CAD build for the part. Positions are in the model's coordinates, mm. A direction names the side the tool comes from. Give positions to 0.01 mm unless a question says otherwise; leave off trailing zeros. Order: outer loops, then holes, each group sorted by start corner. A loop starts at its lowest first (then second) coordinate and runs counter-clockwise, first axis right, second up. Notation, with made-up numbers: (45.5, 54) -> (63.5, 54) arc R21 ccw to (63.5, 87) -> close; hole circle Ø6 at (14, 67.5). An arc over 180 degrees is marked (long way). Answer as CSV lines item,"result".
```python
from build123d import *

# Parameters (mm, degrees)
PAD002_DEPTH    = 25
SKETCH003_R     = 1.1
SKETCH003_W     = 25
SKETCH003_H     = 10
POCKET_DEPTH    = 5
PAD015_DEPTH    = 20
SKETCH029_R     = 1.65
SKETCH029_W     = 23.5
SKETCH029_H     = 12
POCKET009_DEPTH = 50


with BuildPart() as part:
    # Sketch002 → Pad002 (new body)
    with BuildSketch(Plane.XY):
        Polygon((100, 33), (100, 43), (98, 43), (0, 43), (0, 0), (3, 0), (3, 40), (85.5, 28), (85.5, 40), (98, 40), (98, -20), (100, -20), (100, 31), (103.5, 31), (103.5, 43), (102.3, 43), (102.3, 33), align=None)
    extrude(amount=PAD002_DEPTH)

    # Sketch003 → Pocket (cut)
    with BuildSketch(Plane.YZ):
        with Locations((2, 23)):
            Circle(SKETCH003_R)
        with Locations((2, 2)):
            Circle(SKETCH003_R)
        with Locations((14.5, 23)):
            Circle(SKETCH003_R)
        with Locations((14.5, 2)):
            Circle(SKETCH003_R)
        with Locations((12.5, 12.5)):
            Rectangle(SKETCH003_W, SKETCH003_H)
    extrude(amount=POCKET_DEPTH, mode=Mode.SUBTRACT)

    # Sketch018 → Pad015 (join)
    with BuildSketch(Plane.XZ):
        Polygon((100, 0), (100, -103), (83.5, -103), (83.5, -89), (85.5, -89), (85.5, -101), (98, -101), (98, 0), align=None)
    extrude(amount=PAD015_DEPTH)

    # Sketch029 → Pocket009 (cut)
    with BuildSketch(Plane.XY):
        with Locations((54.956858, 34.491576)):
            Circle(SKETCH029_R)
        with Locations((82.956858, 34.491576)):
            Circle(SKETCH029_R)
        with Locations((68.956858, 34.491576)):
            Rectangle(SKETCH029_W, SKETCH029_H)
    extrude(amount=POCKET009_DEPTH, mode=Mode.SUBTRACT)


solid = part.part
```
1) Band-saw the part on C-C, the plane x = 92. Write the cut outline in (y, z), then the cut area to 3 significant figures.
Data:
outline,"(-20, -103) -> (0, -103) -> (0, -101) -> (-20, -101) -> close; (40, 0) -> (43, 0) -> (43, 25) -> (40, 25) -> close"
area,"115 mm2"
2) Band-saw the part on B-B, the plane z = -90.5. Write the cut outline in (x, y).
Data:
outline,"(83.5, -20) -> (85.5, -20) -> (85.5, 0) -> (83.5, 0) -> close; (98, -20) -> (100, -20) -> (100, 0) -> (98, 0) -> close"
3) Band-saw the part on A-A, the plane y = 38. Write the cut outline in (x, z), then the cut area to 3 significant figures.
Data:
outline,"(0, 0) -> (3, 0) -> (3, 25) -> (0, 25) -> close; (16.75, 0) -> (57.21, 0) -> (57.21, 25) -> (16.75, 25) -> close; (80.71, 0) -> (85.5, 0) -> (85.5, 25) -> (80.71, 25) -> close; (98, 0) -> (100, 0) -> (100, 25) -> (98, 25) -> close; (102.3, 0) -> (103.5, 0) -> (103.5, 25) -> (102.3, 25) -> close"
area,"1,290 mm2"
4) Which spindle directions (+Z, -Z, +X, -X, +Y, -Y) get a long thin tool onto all of the face, cutting with end or side? Do faces 1 (the flat face through (69, 40.492, 12)), 2 (the flat face through (98, -3, -25)), 3 (the flat face through (99, 0, -55)), 4 (the flat face through (1, 0, 21)). Say none if no direction does.
Data:
face 1,"+Z, -Z, -Y"
face 2,"+Z, -Y"
face 3,"-Z, +X, -X, +Y"
face 4,"+Z, -Z, -X, -Y"
5) Wall check: line 1 along Z through (x, y) = (2.35, 14.5); line 2 along Y through (x, z) = (2, 23); line 3 along X through (y, z) = (11, 6). Give the ranges that are in metal, low to high. Write a range as [from, to].
Data:
line 1,"z = [0, 0.9], [3.1, 7.5], [17.5, 21.9], [24.1, 25]"
line 2,"y = [0, 0.9], [3.1, 13.4], [15.6, 43]"
line 3,"x = [0, 3], [98, 100]"
6) Pull direction Z, two halves, no side cores. Call faces 5 (the flat face through (103.5, 37, 12)), 6 (the flat face through (1, 12, 7.5)), 7 (the flat face through (36, 37, 25)): pulls with the +Z half, pulls with the -Z half, needs draft (parallel to the pull), parting line crosses it, or undercut.
Data:
face 5,"needs draft"
face 6,"undercut"
face 7,"pulls with the +Z half"
7) Band-saw the part on D-D, the plane y = -14. Write the cut outline in (x, z), then the cut area to 3 significant figures.
Data:
outline,"(83.5, -103) -> (100, -103) -> (100, 25) -> (98, 25) -> (98, -101) -> (85.5, -101) -> (85.5, -89) -> (83.5, -89) -> close"
area,"309 mm2"
8) Pin check, flat tips, straight feed: P1, Ø5, axis at y = 37.5, z = 9, coming from the -X side; P2, Ø7.5, axis at y = 15.5, z = 8, coming from the +X side; P3, Ø0.9, axis at x = 1.5, z = 13, coming from the -Y side; P4, Ø14, axis at x = 90.5, y = -11.5, coming from the +Z side. Stop position of each tip, or through.
Data:
P1,"stops at x = 0"
P2,"stops at x = 100"
P3,"stops at y = 25"
P4,"stops at z = -89"
